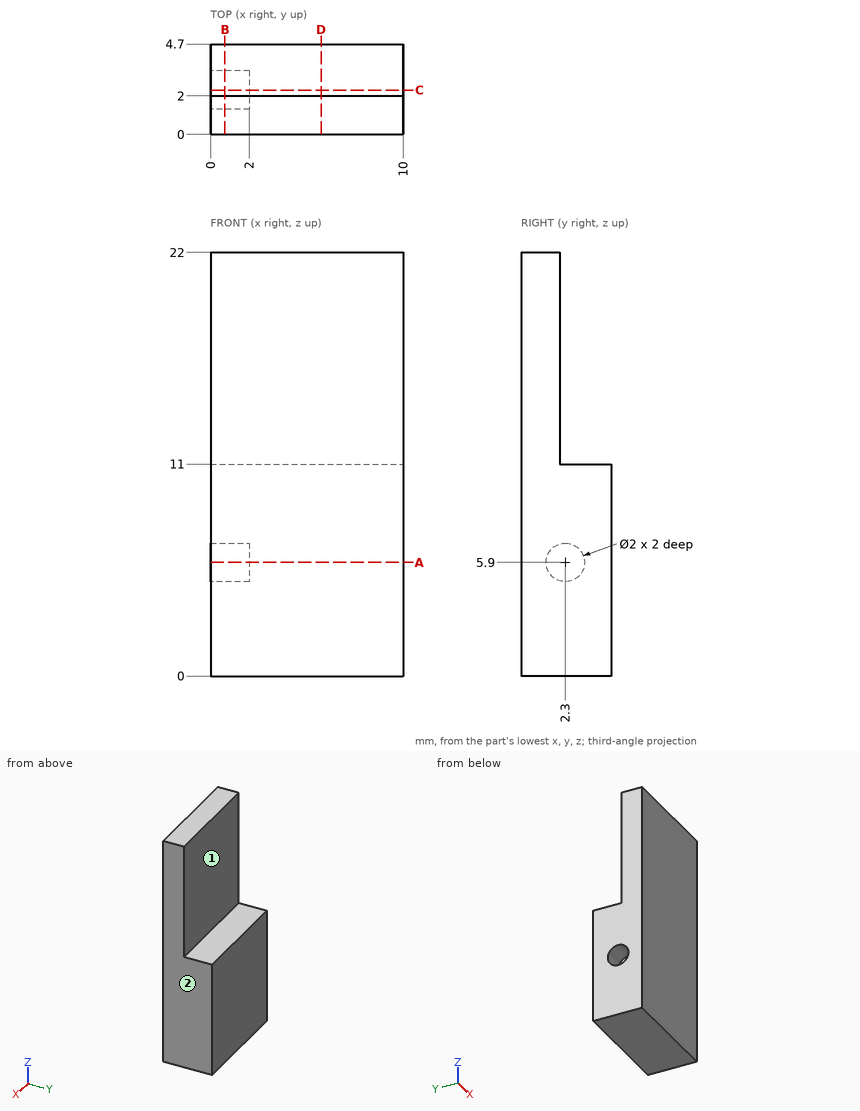
Part print with two shaded views. Sizes in mm from the minimum x, y, z corner. A direction names the side the tool comes from. Coordinates: 2 decimals unless noted, no trailing zeros. Write each loop counter-clockwise with the first axis right and the second up, starting at its lowest first coordinate (ties: lowest second). Pieces come first, ordered by that corner, then holes. Notation, with made-up numbers: (47, -36) - (94, -36) arc R10 ccw to (94, -19) - close; hole circle Ø6 at (81.25, -25.5). An arc over 180 degrees is marked (long way). One line per item, written item: value. Start each with the question number.
1. Slice it at A-A (z = 5.9). Write the cut outline in (x, y).
2. Slice it at D-D (x = 5.75). Write the cut outline in (y, z), plus the area to 3 significant figures.
3. Slice it at C-C (y = 2.3). Write the cut outline in (x, z).
4. Tool access for the marked faces 1 and 2: list every direction of +Z, -Z, +X, -X, +Y, -Y with a clear straight run to the whole face (end or side of a thin tool).
5. Flat gauge pin, fed straight in: pin 1 (1.4 mm diameter, centred on x = 7, y = 3, fed in from +Z). Where does the tip first touch, or does it go through?
6. Slice it at B-B (x = 0.75). Write the cut outline in (y, z).
7. Probe line 1 (Y direction, x = 1.2, z = 5.9); line 2 (Z direction, x = 8.5, y = 4); line 3 (Y direction, x = 8.25, z = 19.75). List the from-to ranges inside material, lowest first. Write a range as from..to.
Answers below:
1. outline: (0, 0) - (10, 0) - (10, 4.7) - (0, 4.7) - (0, 3.3) - (2, 3.3) - (2, 1.3) - (0, 1.3) - close
2. outline: (0, 0) - (4.7, 0) - (4.7, 11) - (2, 11) - (2, 22) - (0, 22) - close
2. area: 73.7 mm^2
3. outline: (0, 0) - (10, 0) - (10, 11) - (0, 11) - (0, 6.9) - (2, 6.9) - (2, 4.9) - (0, 4.9) - close
4. face 1: +Z, +X, -X, +Y
4. face 2: +Z, -Z, +X, +Y, -Y
5. pin 1: stops at z = 11
6. outline: (0, 0) - (4.7, 0) - (4.7, 11) - (2, 11) - (2, 22) - (0, 22) - close; hole circle Ø2 at (2.3, 5.9)
7. line 1: y = 0..1.3, 3.3..4.7
7. line 2: z = 0..11
7. line 3: y = 0..2
